Model file for the job. Use its own axes, mm. A direction names the side the tool comes from. Round coordinates to 2 decimals unless told otherwise and drop trailing zeros. Loops run counter-clockwise (first coordinate to the right, second up) from the corner with the lowest first, then second, coordinate; pieces in that order, holes last. Notation, with made-up numbers: M 53.25,32.5 L 98.25,32.5 A19 ccw 98.25,37.5 Z; hole C -8,88 d8. An arc over 180 degrees is marked long. Answer in a Markdown table with one row per item.
from build123d import *

# Parameters (mm, degrees)
F0_R     = 4
F0_R_2   = 3
F1_DEPTH = 40
F3_R     = 3
F4_DEPTH = 2
F5_R     = 1


with BuildPart() as f1:
    # F0 (on Front) → F1 (new body)
    with BuildSketch(Plane.XZ):
        Circle(F0_R)
        Circle(F0_R_2, mode=Mode.SUBTRACT)
    extrude(amount=F1_DEPTH)

    # F3 (on offset) → F4 (join)
    with BuildSketch(Plane.XZ.offset(25)):
        with BuildLine():
            Line((-7, 0), (-7, -12))
            ThreePointArc((-7, -12), (0, -19), (7, -12))
            Line((7, -12), (7, 0))
            ThreePointArc((7, 0), (0, 7), (-7, 0))
        make_face()
        with Locations((0, -12)):
            Circle(F3_R, mode=Mode.SUBTRACT)
    extrude(amount=F4_DEPTH)

    # F5
    f5_edges = [f1.edges().sort_by_distance(p)[0] for p in [
        (-4, -27, 0),
        (-4, -25, 0),
    ]]
    fillet(f5_edges, radius=F5_R)


solid = f1.part
1. Saw through at D-D (y = -27.5). Write the cut outline in (x, z), and give its area (3 significant figures).
Verdict:
| item | result |
|---|---|
| outline | C 0,0 d8.27; hole C 0,0 d6 |
| area | 25.4 mm² |
2. Pin check, flat tips, straight feed: pin 1 (1.5 mm diameter, centred on x = 0, z = 1.5, fed in from -Y); pin 2 (4 mm diameter, centred on x = -4.5, y = -23.5, fed in from +Z); pin 3 (5 mm diameter, centred on x = 0, z = -12, fed in from -Y); pin 4 (10 mm diameter, centred on y = -33.5, z = 3, fed in from +X). Stop position of each tip, or through.
Verdict:
| item | result |
|---|---|
| pin 1 | stops at y = -27 |
| pin 2 | stops at z = 6.24 |
| pin 3 | passes through |
| pin 4 | stops at x = 4 |
3. Tool access for faces 1 (the cylindrical face through (-3, -12, 0)), 2 (the cylindrical face through (-0.867, -33.916, -3.905)), 3 (the cylindrical face through (0, -26, 7)): list every direction of +Z, -Z, +X, -X, +Y, -Y with a clear straight run to the whole face (end or side of a thin tool).
Verdict:
| item | result |
|---|---|
| face 1 | +Y |
| face 2 | -Y |
| face 3 | +Z, +Y, -Y |
4. Wall check: probe 1 along X at (y, z) = (-8.5, 0); probe 2 along Z at (x, y) = (0, -25.9); probe 3 along Z at (x, y) = (-1.5, -12). Give the ranges that are in metal, low to high.
Verdict:
| item | result |
|---|---|
| probe 1 | x = -4 to -3, 3 to 4 |
| probe 2 | z = -19 to -15, -9 to 7 |
| probe 3 | z = -3.71 to -2.6, 2.6 to 3.71 |
5. Mould opens along X. For faces 4 (the cylindrical face through (0, -26, -19)), 5 (the flat face through (0, -25, -6)), 6 (the cylindrical face through (-3, -33, 0)) say: +X half, -X half, draft (parallel to the pull), parting line (faces both ways), or undercut.
Verdict:
| item | result |
|---|---|
| face 4 | parting line |
| face 5 | draft |
| face 6 | undercut |
6. Saw through at A-A (x = 0). Write the cut outline in (y, z), and give its area (3 significant figures).
Verdict:
| item | result |
|---|---|
| outline | M -40,-4 L -28,-4 A1 cw -27,-5 L -27,-9 L -25,-9 L -25,-5 A1 cw -24,-4 L 0,-4 L 0,-3 L -25,-3 L -25,3 L 0,3 L 0,4 L -24,4 A1 cw -25,5 L -25,7 L -27,7 L -27,5 A1 cw -28,4 L -40,4 L -40,3 L -27,3 L -27,-3 L -40,-3 Z; M -27,-19 L -25,-19 L -25,-15 L -27,-15 Z |
| area | 117 mm² |
7. Saw through at B-B (y = -15.5). Write the cut outline in (x, z).
Verdict:
| item | result |
|---|---|
| outline | C 0,0 d8; hole C 0,0 d6 |
8. Saw through at C-C (z = -7.5). Write the cut outline in (x, y).
Verdict:
| item | result |
|---|---|
| outline | M -7,-27 L 7,-27 L 7,-25 L -7,-25 Z |
